```python
from build123d import *

# Parameters (mm, degrees)
PAD_DEPTH       = 2
PAD001_DEPTH    = 5.4
SKETCH002_W     = 26
SKETCH002_H     = 3.75
SKETCH002_H_2   = 1.75
SKETCH002_W_2   = 12
SKETCH002_H_3   = 25
PAD002_DEPTH    = 3
PAD003_DEPTH    = 2.4
PAD005_DEPTH    = 7.9
SKETCH007_W     = 5
SKETCH007_H     = 1.5
POCKET001_DEPTH = 1.2
SKETCH008_W     = 5
SKETCH008_H     = 1.5
POCKET002_DEPTH = 1.2
SKETCH009_W     = 10
SKETCH009_H     = 2
POCKET003_DEPTH = 1.8
SKETCH020_W     = 5
SKETCH020_H     = 1.5
POCKET009_DEPTH = 1.2
SKETCH021_W     = 2
SKETCH021_H     = 15
PAD010_DEPTH    = 1.5


with BuildPart() as part:
    # Sketch → Pad (new body)
    with BuildSketch(Plane.XY):
        with BuildLine():
            Line((149.26, 103.29), (149.26, 4))
            ThreePointArc((145.26, 0), (148.088427, 1.171573), (149.26, 4))
            Line((4, 0), (145.26, 0))
            ThreePointArc((0, 4), (1.171573, 1.171573), (4, 0))
            Line((0, 103.29), (0, 4))
            ThreePointArc((4, 107.29), (1.171573, 106.118427), (0, 103.29))
            Line((4, 107.29), (145.26, 107.29))
            ThreePointArc((149.26, 103.29), (148.088427, 106.118427), (145.26, 107.29))
        make_face()
    extrude(amount=PAD_DEPTH)

    # Sketch001 (on Face10 of Pad) → Pad001 (join)
    with BuildSketch(Plane.XY.offset(2)):
        with BuildLine():
            ThreePointArc((4, 107.29), (1.171573, 106.118427), (0, 103.29))
            Line((0, 4), (0, 103.29))
            ThreePointArc((0, 4), (1.171573, 1.171573), (4, 0))
            Line((145.26, 0), (4, 0))
            ThreePointArc((145.26, 0), (148.088427, 1.171573), (149.26, 4))
            Line((149.26, 103.29), (149.26, 4))
            ThreePointArc((149.26, 103.29), (148.088427, 106.118427), (145.26, 107.29))
            Line((4, 107.29), (145.26, 107.29))
        make_face()
        with BuildLine():
            Line((4, 105.49), (145.26, 105.49))
            ThreePointArc((147.46, 103.289998), (146.815636, 104.845634), (145.26, 105.49))
            Line((147.46, 103.289998), (147.46, 3.999998))
            ThreePointArc((145.259998, 1.8), (146.815633, 2.444364), (147.46, 3.999998))
            Line((145.259998, 1.8), (3.999998, 1.8))
            ThreePointArc((1.8, 4), (2.444364, 2.444366), (3.999998, 1.8))
            Line((1.8, 4), (1.8, 103.29))
            ThreePointArc((4, 105.49), (2.444365, 104.845635), (1.8, 103.29))
        make_face(mode=Mode.SUBTRACT)
    extrude(amount=PAD001_DEPTH)

    # Sketch002 (on Face10 of Pad001) → Pad002 (join)
    with BuildSketch(Plane.XY.offset(2)):
        with Locations((53, 24.925)):
            Rectangle(SKETCH002_W, SKETCH002_H)
        with Locations((53, 2.675)):
            Rectangle(SKETCH002_W, SKETCH002_H_2)
        with Locations((34, 14.3)):
            Rectangle(SKETCH002_W_2, SKETCH002_H_3)
    extrude(amount=PAD002_DEPTH)

    # Sketch003 (on Face21 of Pad002) → Pad003 (join)
    with BuildSketch(Plane.XY.offset(5)):
        Polygon((28, 1.8), (28, 26.8), (66, 26.8), (66, 24.8), (40, 24.8), (40, 1.8), align=None)
    extrude(amount=PAD003_DEPTH)

    # Sketch006 (on Face22 of Pad003) → Pad005 (join)
    with BuildSketch(Plane.XY.offset(2)):
        with BuildLine():
            ThreePointArc((1.8, 4), (2.444364, 2.444366), (3.999998, 1.8))
            Line((3.999998, 1.8), (28, 1.8))
            Line((28, 1.8), (28, 3.55))
            Line((28, 3.55), (3.55, 3.55))
            Line((3.55, 3.55), (3.55, 103.74))
            Line((3.55, 103.74), (121.46, 103.74))
            Line((121.46, 103.74), (121.46, 105.49))
            Line((121.46, 105.49), (3.999988, 105.49))
            ThreePointArc((3.999988, 105.49), (2.444361, 104.845631), (1.8, 103.29))
            Line((1.8, 103.29), (1.8, 4))
        make_face()
        with BuildLine():
            ThreePointArc((145.259998, 1.8), (146.815633, 2.444364), (147.46, 3.999997))
            Line((147.46, 63.55), (147.46, 3.999997))
            Line((145.71, 63.55), (147.46, 63.55))
            Line((145.71, 63.55), (145.71, 3.55))
            Line((66, 3.55), (145.71, 3.55))
            Line((66, 1.8), (66, 3.55))
            Line((145.259998, 1.8), (66, 1.8))
        make_face()
    extrude(amount=PAD005_DEPTH)

    # Sketch007 (on Face11 of Pad005) → Pocket001 (cut)
    with BuildSketch(Plane(origin=(1.8, 0, 0), x_dir=(0, -1, 0), z_dir=(-1, 0, 0))):
        with Locations((-95.99, 8.15)):
            Rectangle(SKETCH007_W, SKETCH007_H)
        with Locations((-11.3, 8.15)):
            Rectangle(SKETCH007_W, SKETCH007_H)
    extrude(amount=-POCKET001_DEPTH, mode=Mode.SUBTRACT)

    # Sketch008 (on Face38 of Pocket001) → Pocket002 (cut)
    with BuildSketch(Plane.YZ.offset(147.46)):
        with Locations((11.3, 8.15)):
            Rectangle(SKETCH008_W, SKETCH008_H)
        with Locations((56.3, 8.15)):
            Rectangle(SKETCH008_W, SKETCH008_H)
    extrude(amount=-POCKET002_DEPTH, mode=Mode.SUBTRACT)

    # Sketch009 (on Face4 of Pocket002) → Pocket003 (cut)
    with BuildSketch(Plane.YZ.offset(149.26)):
        with Locations((78.29, 6.4)):
            Rectangle(SKETCH009_W, SKETCH009_H)
    extrude(amount=-POCKET003_DEPTH, mode=Mode.SUBTRACT)

    # Sketch020 (on Face17 of Pocket003) → Pocket009 (cut)
    with BuildSketch(Plane(origin=(0, 105.49, 0), x_dir=(-1, 0, 0), z_dir=(0, 1, 0))):
        with Locations((-111.96, 8.15)):
            Rectangle(SKETCH020_W, SKETCH020_H)
    extrude(amount=-POCKET009_DEPTH, mode=Mode.SUBTRACT)

    # Sketch021 (on Face16 of Pocket009) → Pad010 (join)
    with BuildSketch(Plane.XY.offset(2)):
        with Locations((144.46, 78.29)):
            Rectangle(SKETCH021_W, SKETCH021_H)
    extrude(amount=PAD010_DEPTH)


solid = part.part
```
Geometry: final body of the model. Coordinates: model frame, mm. A direction names the side the tool comes from. Coordinates: 2 decimals unless noted, no trailing zeros. Loops run counter-clockwise (first coordinate to the right, second up) from the corner with the lowest first, then second, coordinate; pieces in that order, holes last. Notation, with made-up numbers: M 24,70 L 40,70 A20 ccw 40,109 Z; hole C 53.25,-28 d7. An arc over 180 degrees is marked long. Put each result on its own line as item: value.
(1) Cut plane B-B on x = 35. Return the cut outline in (y, z), then the cut area to 3 significant figures.
Answer sheet:
outline: M 0,0 L 107.29,0 L 107.29,7.4 L 105.49,7.4 L 105.49,9.9 L 103.74,9.9 L 103.74,2 L 26.8,2 L 26.8,7.4 L 0,7.4 Z
area: 383 mm^2
(2) Cut plane D-D on y = 21. Return the cut outline in (x, z), then the cut area to 3 significant figures.
Answer sheet:
outline: M 0,0 L 149.26,0 L 149.26,7.4 L 147.46,7.4 L 147.46,9.9 L 145.71,9.9 L 145.71,2 L 40,2 L 40,7.4 L 28,7.4 L 28,2 L 3.55,2 L 3.55,9.9 L 1.8,9.9 L 1.8,7.4 L 0,7.4 Z
area: 410 mm^2
(3) Draft query along X for faces 3 (the face through (104, 3.55, 6)), 4 (the face through (148.119, 106.087, 3.648)), 5 (the face through (76, 0, 4)). Return one class per face: pulls with the +X half, pulls with the -X half, needs draft (parallel to the pull), parting line crosses it, or undercut.
Answer sheet:
face 3: undercut
face 4: pulls with the +X half
face 5: needs draft
(4) First-contact query: pin 1 (1.9 mm diameter, centred on x = 54, y = 3, fed in from +Z); pin 2 (1.2 mm diameter, centred on x = 117.5, z = 9, fed in from -Y); pin 3 (1 mm diameter, centred on x = 144.5, y = 79.5, fed in from +Z). Flat tips, straight axial feed; report the tip coordinate or a pass-through.
Answer sheet:
pin 1: stops at z = 5
pin 2: stops at y = 1.8
pin 3: stops at z = 3.5
(5) Cut plane A-A on y = 57. Return the cut outline in (x, z), then the cut area to 3 significant figures.
Answer sheet:
outline: M 0,0 L 149.26,0 L 149.26,7.4 L 146.26,7.4 L 146.26,8.9 L 147.46,8.9 L 147.46,9.9 L 145.71,9.9 L 145.71,2 L 3.55,2 L 3.55,9.9 L 1.8,9.9 L 1.8,7.4 L 0,7.4 Z
area: 344 mm^2
(6) Access query for faces 1 (the face through (53, 23.05, 3)), 2 (the face through (1.141, 1.203, 3.648)). Directions: +Z, -Z, +X, -X, +Y, -Y. A direction counts if a zero-diameter tool reaches every point of the face in a straight line with its end or side. Return the directions, or none.
Answer sheet:
face 1: +Z
face 2: +Z, -Z, -X, -Y
(7) Material intervals for probe 1 along X at (y, z) = (24, 3.75); probe 2 along X at (y, z) = (14.5, 3.25); probe 3 along X at (y, z) = (99, 6.5), sorted ascending.
Answer sheet:
probe 1: x = 0 to 3.55, 28 to 66, 145.71 to 149.26
probe 2: x = 0 to 3.55, 28 to 40, 145.71 to 149.26
probe 3: x = 0 to 3.55, 147.46 to 149.26
(8) Cut plane C-C on x = 83.5. Return the cut outline in (y, z), then the cut area to 3 significant figures.
Answer sheet:
outline: M 0,0 L 107.29,0 L 107.29,7.4 L 105.49,7.4 L 105.49,9.9 L 103.74,9.9 L 103.74,2 L 3.55,2 L 3.55,9.9 L 1.8,9.9 L 1.8,7.4 L 0,7.4 Z
area: 262 mm^2
